Verification items for this drawing (mm, ordinates from the low corner). Coordinates: 2 decimals unless noted, no trailing zeros. Order: outer loops, then holes, each group sorted by start corner. A loop starts at its lowest first (then second) coordinate and runs counter-clockwise, first axis right, second up. Notation, with made-up numbers: (1.25, 3) -> (36.25, 3) arc R24 cw to (36.25, 18) -> close; hole circle Ø3 at (-9.75, 42.5). An arc over 180 degrees is marked (long way). Write item = value, one per line. Start each with the question number.
1. Thickness scan on line 1 along Y through (x, z) = (30, 7.5) (3 decimals); line 2 along Y through (x, z) = (28.5, 4.5); line 3 along X through (y, z) = (17.5, 11.75). Record the ranges inside material, lowest first. Write a range as from..to.
2. Cross-section at A-A on x = 30. Record the cut outline in (y, z) (3 decimals).
3. Cross-section at D-D on y = 23. Record the cut outline in (x, z).
4. Release check for a two-part mould opening along X. For the marked faces 1, 2, 3 and 4 record: +X half, -X half, draft (parallel to the pull), parting line (faces both ways), or undercut.
5. Go/stop test with flat-tipped pins: P1, Ø1, axis at y = 30.5, z = 10, coming from the +X side; P2, Ø1, axis at y = 34, z = 9.5, coming from the +X side; P3, Ø2, axis at x = 45.5, z = 6, coming from the +Y side; P4, Ø8.5, axis at x = 30, y = 10, coming from the +Z side. Record where each tip stops, or that it passes through.
6. Cross-section at B-B on z = 6.25. Record the cut outline in (x, y) (3 decimals), plus the area to 3 significant figures.
7. Cross-section at C-C on x = 6. Record the cut outline in (y, z), plus the area to 3 significant figures.
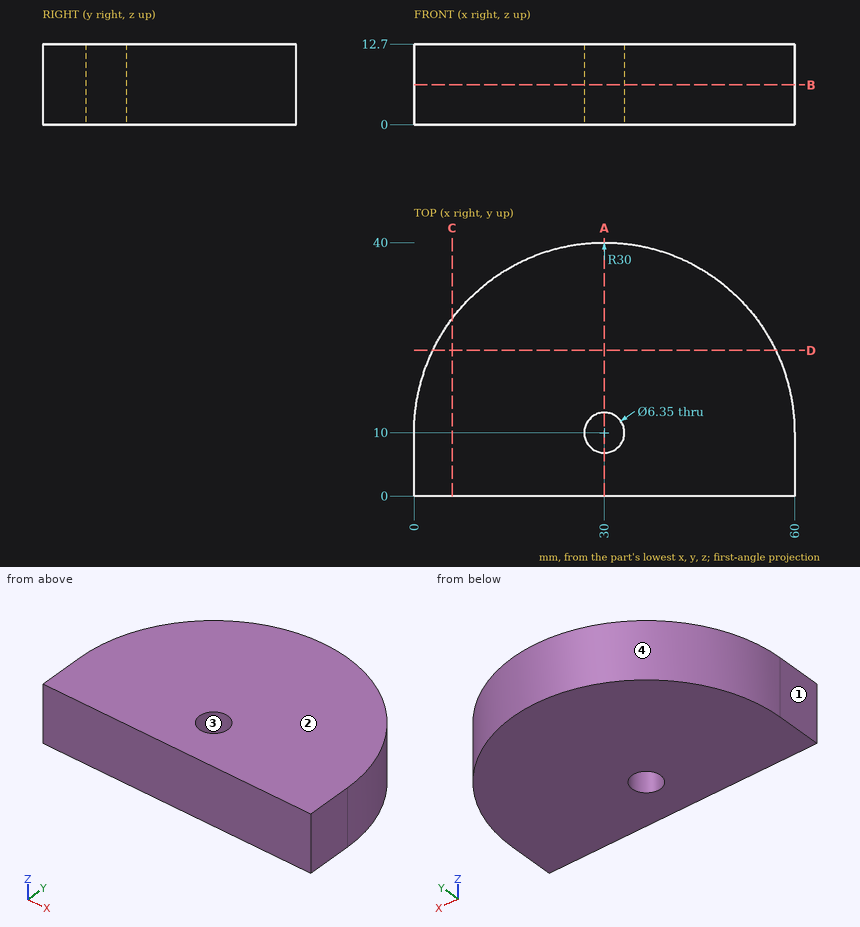
Worked out:
q1.line_1 = 0..6.825, 13.175..40
q1.line_2 = 0..7.2, 12.8..39.96
q1.line_3 = 0.95..59.05
q2.outline = (0, 0) -> (6.825, 0) -> (6.825, 12.7) -> (0, 12.7) -> close; (13.175, 0) -> (40, 0) -> (40, 12.7) -> (13.175, 12.7) -> close
q3.outline = (2.96, 0) -> (57.04, 0) -> (57.04, 12.7) -> (2.96, 12.7) -> close
q4.face_1 = -X half
q4.face_2 = draft
q4.face_3 = undercut
q4.face_4 = parting line
q5.P1 = 52.36
q5.P2 = 48.65
q5.P3 = 36.26
q5.P4 = 12.7
q6.outline = (0, 0) -> (60, 0) -> (60, 10) arc R30 ccw to (0, 10) -> close; hole circle Ø6.35 at (30, 10)
q6.area = 1,980 mm²
q7.outline = (0, 0) -> (28, 0) -> (28, 12.7) -> (0, 12.7) -> close
q7.area = 356 mm²
